```python
from build123d import *
from build123d.topology import SkipClean

# Parameters (mm, degrees)
MODEL_R             = 6.25
BOSS_EXTRUDE1_DEPTH = 2.4
BOSS_EXTRUDE2_START = 3
SKETCH2_R           = 8
SKETCH2_R_2         = 6.25
BOSS_EXTRUDE2_DEPTH = 3


with BuildPart() as part:
    # Model → Boss-Extrude1 (new body)
    with BuildSketch(Plane.XY):
        with BuildLine():
            ThreePointArc((5.219883463, 8.290306898), (5.649962695, 10.449038711), (5.222503822, 12.608290919))
            ThreePointArc((5.222503822, 12.608290919), (3.39344735, 11.383736442), (2.171116571, 9.55319316))
            ThreePointArc((2.171116571, 9.55319316), (7.05e-06, 8.10252753), (-2.171097098, 9.553201202))
            ThreePointArc((-2.171097098, 9.553201202), (-3.393450986, 11.383763689), (-5.222542517, 12.608317574))
            ThreePointArc((-5.222542517, 12.608317574), (-5.649987545, 10.449048181), (-5.219883434, 8.290306876))
            ThreePointArc((-5.219883434, 8.290306876), (-5.729313534, 5.729323511), (-8.290298786, 5.219902898))
            ThreePointArc((-8.290298786, 5.219902898), (-10.449036556, 5.649974072), (-12.608290861, 5.222503812))
            ThreePointArc((-12.608290861, 5.222503812), (-11.383736397, 3.393447352), (-9.553193136, 2.171116571))
            ThreePointArc((-9.553193136, 2.171116571), (-8.102527499, 7.032e-06), (-9.55320119, -2.171097126))
            ThreePointArc((-9.55320119, -2.171097126), (-11.38376367, -3.393451008), (-12.608317555, -5.222542529))
            ThreePointArc((-12.608317555, -5.222542529), (-10.449048162, -5.649987556), (-8.290306857, -5.219883446))
            ThreePointArc((-8.290306857, -5.219883446), (-5.729323474, -5.729313553), (-5.219902867, -8.290298826))
            ThreePointArc((-5.219902867, -8.290298826), (-5.649974041, -10.449036588), (-5.222503789, -12.608290885))
            ThreePointArc((-5.222503789, -12.608290885), (-3.393447328, -11.383736421), (-2.171116547, -9.55319316))
            ThreePointArc((-2.171116547, -9.55319316), (-7.008e-06, -8.102527522), (2.17109715, -9.553201214))
            ThreePointArc((2.17109715, -9.553201214), (3.393451032, -11.383763694), (5.222542552, -12.608317579))
            ThreePointArc((5.222542552, -12.608317579), (5.64998758, -10.449048185), (5.21988347, -8.290306881))
            ThreePointArc((5.21988347, -8.290306881), (5.729313577, -5.729323498), (8.29029885, -5.219902891))
            ThreePointArc((8.29029885, -5.219902891), (10.449036612, -5.649974065), (12.608290909, -5.222503812))
            ThreePointArc((12.608290909, -5.222503812), (11.383736445, -3.393447352), (9.553193184, -2.171116571))
            ThreePointArc((9.553193184, -2.171116571), (8.102527546, -7.031e-06), (9.553201238, 2.171097126))
            ThreePointArc((9.553201238, 2.171097126), (11.383763724, 3.393451015), (12.60831761, 5.222542545))
            ThreePointArc((12.60831761, 5.222542545), (10.449048209, 5.649987575), (8.290306898, 5.219883463))
            ThreePointArc((8.290306898, 5.219883463), (5.729299098, 5.729299098), (5.219883463, 8.290306898))
        make_face()
        Circle(MODEL_R, mode=Mode.SUBTRACT)
    extrude(amount=BOSS_EXTRUDE1_DEPTH)

    # Sketch2 → Boss-Extrude2 (add)
    with SkipClean():  # the faces are left unmerged after this step: merging them gives an invalid solid
        with BuildSketch(Plane(origin=(0, 0, 0), x_dir=(-1, 0, 0), z_dir=(0, 0, -1)).offset(BOSS_EXTRUDE2_START)):
            Circle(SKETCH2_R)
            Circle(SKETCH2_R_2, mode=Mode.SUBTRACT)
        boss_extrude2 = extrude(amount=-BOSS_EXTRUDE2_DEPTH)

    # Mirror1: Boss-Extrude2 across plane
    add(boss_extrude2.mirror(Plane(origin=(0, 0, 1.199999886), x_dir=(1, 0, 0), z_dir=(0, 0, -1))))


solid = part.part
```
CAD build for the part. Positions are in the model's coordinates, mm. A direction names the side the tool comes from. Round coordinates to 2 decimals unless told otherwise and drop trailing zeros. Order: outer loops, then holes, each group sorted by start corner. A loop starts at its lowest first (then second) coordinate and runs counter-clockwise, first axis right, second up.
Item 1: Saw through at C-C on z = 1.75. Write the cut outline in (x, y), then the cut area to 3 significant figures.
Item 2: Mould opens along Y. For faces 1 (the face through (-3.42, -11.41, 1.18)), 2 (the face through (5.76, 5.7, 1.18)), 3 (the face through (1.73, -7.81, 3.92)) say: pulls with the +Y half, pulls with the -Y half, needs draft (parallel to the pull), parting line crosses it, or undercut.
Item 3: Tool access for faces 4 (the face through (-11.41, 3.42, 1.18)), 5 (the face through (-8, -3, 2.4)), 6 (the face through (-8, -3, 0)): list every direction of +Z, -Z, +X, -X, +Y, -Y with a clear straight run to the whole face (end or side of a thin tool).
Item 4: Pin check, flat tips, straight feed: pin 1 (2 mm diameter, centred on y = -2, z = 1, fed in from -X); pin 2 (1 mm diameter, centred on x = -9.5, z = 1.5, fed in from -Y); pin 3 (1 mm diameter, centred on y = -1, z = 2.5, fed in from +X); pin 4 (11 mm diameter, centred on x = 0, y = 0, fed in from -Z). Stop position of each tip, or through.
Item 5: Saw through at A-A on y = 0. Write the cut outline in (x, z).
Item 6: Saw through at D-D on x = -10.5. Write the cut outline in (y, z).
Item 7: Probe line 1 along X through (y, z) = (0, 1.4); line 2 along Y through (x, z) = (0, -1.9). List the from-to ranges inside material, lowest first.
Reported:
1. outline: (-12.61, -5.22) arc R5.65 ccw to (-8.29, -5.22) arc R2.35 cw to (-5.22, -8.29) arc R5.65 ccw to (-5.22, -12.61) arc R5.65 ccw to (-2.17, -9.55) arc R2.35 cw to (2.17, -9.55) arc R5.65 ccw to (5.22, -12.61) arc R5.65 ccw to (5.22, -8.29) arc R2.35 cw to (8.29, -5.22) arc R5.65 ccw to (12.61, -5.22) arc R5.65 ccw to (9.55, -2.17) arc R2.35 cw to (9.55, 2.17) arc R5.65 ccw to (12.61, 5.22) arc R5.65 ccw to (8.29, 5.22) arc R2.35 cw to (5.22, 8.29) arc R5.65 ccw to (5.22, 12.61) arc R5.65 ccw to (2.17, 9.55) arc R2.35 cw to (-2.17, 9.55) arc R5.65 ccw to (-5.22, 12.61) arc R5.65 ccw to (-5.22, 8.29) arc R2.35 cw to (-8.29, 5.22) arc R5.65 ccw to (-12.61, 5.22) arc R5.65 ccw to (-9.55, 2.17) arc R2.35 cw to (-9.55, -2.17) arc R5.65 ccw to start; hole circle Ø12.5 at (0, 0)
1. area: 207 mm2
2. face 1: pulls with the -Y half
2. face 2: undercut
2. face 3: parting line crosses it
3. face 4: +Z, -Z, -X
3. face 5: +Z
3. face 6: -Z
4. pin 1: stops at x = -10.95
4. pin 2: stops at y = -5.63
4. pin 3: stops at x = 8.64
4. pin 4: passes through
5. outline: (-8.1, 0) - (-8, 0) - (-8, -3) - (-6.25, -3) - (-6.25, 5.4) - (-8, 5.4) - (-8, 2.4) - (-8.1, 2.4) - close; (6.25, -3) - (8, -3) - (8, 0) - (8.1, 0) - (8.1, 2.4) - (8, 2.4) - (8, 5.4) - (6.25, 5.4) - close
6. outline: (-5.65, 0) - (-2.67, 0) - (-2.67, 2.4) - (-5.65, 2.4) - close; (2.67, 0) - (5.65, 0) - (5.65, 2.4) - (2.67, 2.4) - close
7. line 1: x = -8.1 to -6.25, 6.25 to 8.1
7. line 2: y = -8 to -6.25, 6.25 to 8
